CAD build for the part. Positions are in the model's coordinates, mm. A direction names the side the tool comes from. Give positions to 0.01 mm unless a question says otherwise; leave off trailing zeros. Order: outer loops, then holes, each group sorted by start corner. A loop starts at its lowest first (then second) coordinate and runs counter-clockwise, first axis right, second up. Notation, with made-up numbers: (39.5, 34.5) -> (65.5, 34.5) arc R15 cw to (65.5, 41.5) -> close; hole circle Ø4 at (-9.75, 54). An arc over 180 degrees is marked (long way). Use one line per item in the form item = value. Start each with the question number.
1) Cut at D-D, the plane x = 169. Give the cut face in (y, z).
2) Mould opens along Y. For faces 1 (the face through (395, -187, 489.296)), 2 (the face through (238, -278, -5.585)) say: pulls with the +Y half, pulls with the -Y half, needs draft (parallel to the pull), parting line crosses it, or undercut.
3) Cut at A-A, the plane z = 162. Give the cut face in (x, y), and give its area (3 significant figures).
4) Cut at B-B, the plane y = -51. Give the cut face in (x, z).
5) Tool access for faces 3 (the face through (49, -31, 22.261)), 4 (the face through (498.351, -326, 260)), 5 (the face through (235, -186, 564.415)): list every direction of +Z, -Z, +X, -X, +Y, -Y with a clear straight run to the whole face (end or side of a thin tool).
6) Drop flat-ended pins along their axis: P1, Ø10, axis at x = 100.5, z = 456, coming from the -Y side; P2, Ø10.5, axis at x = 473, z = 203.5, coming from the +Y side; P3, Ø3, axis at x = 220, z = 343, coming from the +Y side. Give the stop position or say it passes through.
7) Probe line 1 (X direction, y = -195, z = 46.5); line 2 (X direction, y = -248, z = 331); line 3 (X direction, y = -18, z = 507). List the from-to ranges inside material, lowest first.
8) Cut at C-C, the plane x = 60.5. Give the cut face in (y, z), and give its area (3 significant figures).
from build123d import *

# Parameters (mm, degrees)
F0_W      = 524
F0_H      = 604
F0_W_2    = 520
F0_H_2    = 600
F1_DEPTH  = 340
F2_W      = 310
F2_H      = 240
F2_W_2    = 180
F2_H_2    = 110
F2_H_3    = 5
F3_DEPTH  = 600
F2_W_3    = 65
F2_H_4    = 307.9086494446
F4_DEPTH  = 600
F5_DEPTH  = 600
F6_W      = 182.5336068869
F6_H      = 90
F7_DEPTH  = 70
F8_W      = 180
F8_H      = 29.6823031265
F9_DEPTH  = 110
F10_W     = 62.9086494446
F10_H     = 155
F11_DEPTH = 70
F12_DEPTH = 380
F13_W     = 110
F13_H     = 75
F14_DEPTH = 140
F15_W     = 110
F15_H     = 75.1196961854
F16_DEPTH = 140


with BuildPart() as f1:
    # F0 (on Front) → F1 (new body)
    with BuildSketch(Plane.XZ):
        with Locations((238.3513055446, 264.4152384256)):
            Rectangle(F0_W, F0_H)
        with Locations((238.3513055446, 264.4152384256)):
            Rectangle(F0_W_2, F0_H_2, mode=Mode.SUBTRACT)
    extrude(amount=F1_DEPTH)

    # F2 (on face) → F3 (join)
    with BuildSketch(Plane.XY.offset(-35.5847615744)):
        Polygon((-21.6486944554, -307.9086494446), (-21.6486944554, -312.9086494446), (498.3513055446, -312.9086494446), (498.3513055446, -307.9086494446), (463.3513055446, -307.9086494446), (398.3513055446, -307.9086494446), (393.3513055446, -307.9086494446), (83.3513055446, -307.9086494446), (78.3513055446, -307.9086494446), (13.3513055446, -307.9086494446), align=None)
        with Locations((238.3513055446, -187.9086494446)):
            Rectangle(F2_W, F2_H)
        with Locations((238.3513055446, -187.9086494446)):
            Rectangle(F2_W_2, F2_H_2, mode=Mode.SUBTRACT)
        with Locations((238.3513055446, -65.4086494446)):
            Rectangle(F2_W, F2_H_3)
    extrude(amount=F3_DEPTH)

    # F2 (on face) → F4 (join)
    with BuildSketch(Plane.XY.offset(-35.5847615744)):
        with Locations((45.8513055446, -153.9543247223)):
            Rectangle(F2_W_3, F2_H_4)
        with Locations((430.8513055446, -153.9543247223)):
            Rectangle(F2_W_3, F2_H_4)
    extrude(amount=F4_DEPTH)

    # F2 (on face) → F5 (join)
    with BuildSketch(Plane.XY.offset(-35.5847615744)):
        Polygon((78.3513055446, 0), (78.3513055446, -307.9086494446), (83.3513055446, -307.9086494446), (83.3513055446, -67.9086494446), (83.3513055446, -62.9086494446), (83.3513055446, 0), align=None)
        Polygon((393.3513055446, -307.9086494446), (398.3513055446, -307.9086494446), (398.3513055446, 0), (393.3513055446, 0), (393.3513055446, -62.9086494446), (393.3513055446, -67.9086494446), align=None)
    extrude(amount=F5_DEPTH)

    # F6 (on face) → F7 (cut)
    with BuildSketch(Plane.XZ.offset(312.9086494446)):
        with Locations((239.1115501523, 39.4152384256)):
            Rectangle(F6_W, F6_H)
    extrude(amount=-F7_DEPTH, mode=Mode.SUBTRACT)

    # F8 (on face) → F9 (join)
    with BuildSketch(Plane.XZ.offset(132.9086494446)):
        with Locations((238.3513055446, -20.7436100112)):
            Rectangle(F8_W, F8_H)
    extrude(amount=F9_DEPTH)

    # F10 (on face) → F11 (cut)
    with BuildSketch(Plane(origin=(393.3513055446, 0, 0), x_dir=(0, -1, 0), z_dir=(-1, 0, 0))):
        with Locations((31.4543247223, 99.7613327205)):
            Rectangle(F10_W, F10_H)
    extrude(amount=-F11_DEPTH, mode=Mode.SUBTRACT)

    # F10 (on face) → F12 (cut)
    with BuildSketch(Plane(origin=(393.3513055446, 0, 0), x_dir=(0, -1, 0), z_dir=(-1, 0, 0))):
        with Locations((31.4543247223, 99.7613327205)):
            Rectangle(F10_W, F10_H)
    extrude(amount=F12_DEPTH, mode=Mode.SUBTRACT)

    # F13 (on face) → F14 (cut)
    with BuildSketch(Plane.YZ.offset(148.3513055446)):
        with Locations((-187.9086494446, 526.9152384256)):
            Rectangle(F13_W, F13_H)
    extrude(amount=-F14_DEPTH, mode=Mode.SUBTRACT)

    # F15 (on face) → F16 (cut)
    with BuildSketch(Plane(origin=(328.3513055446, 0, 0), x_dir=(0, -1, 0), z_dir=(-1, 0, 0))):
        with Locations((187.9086494446, 526.8553903329)):
            Rectangle(F15_W, F15_H)
    extrude(amount=-F16_DEPTH, mode=Mode.SUBTRACT)


solid = f1.part
Result:
q1.outline = (-340, -37.58) -> (0, -37.58) -> (0, -35.58) -> (-62.91, -35.58) -> (-62.91, 564.42) -> (0, 564.42) -> (0, 566.42) -> (-340, 566.42) -> (-340, 564.42) -> (-312.91, 564.42) -> (-312.91, 84.42) -> (-242.91, 84.42) -> (-242.91, 564.42) -> (-132.91, 564.42) -> (-132.91, -5.9) -> (-242.91, -5.9) -> (-242.91, -5.58) -> (-312.91, -5.58) -> (-312.91, -35.58) -> (-340, -35.58) -> close
q2.face_1 = undercut
q2.face_2 = needs draft
q3.outline = (-23.65, -340) -> (-21.65, -340) -> (-21.65, -312.91) -> (498.35, -312.91) -> (498.35, -340) -> (500.35, -340) -> (500.35, 0) -> (498.35, 0) -> (498.35, -307.91) -> (463.35, -307.91) -> (463.35, -62.91) -> (13.35, -62.91) -> (13.35, -307.91) -> (-21.65, -307.91) -> (-21.65, 0) -> (-23.65, 0) -> close; hole (148.35, -242.91) -> (328.35, -242.91) -> (328.35, -132.91) -> (148.35, -132.91) -> close
q3.area = 94,400 mm²
q4.outline = (-23.65, -37.58) -> (500.35, -37.58) -> (500.35, 566.42) -> (-23.65, 566.42) -> close; hole (-21.65, -35.58) -> (13.35, -35.58) -> (13.35, 22.26) -> (83.35, 22.26) -> (83.35, -35.58) -> (393.35, -35.58) -> (393.35, 22.26) -> (463.35, 22.26) -> (463.35, -35.58) -> (498.35, -35.58) -> (498.35, 564.42) -> (463.35, 564.42) -> (463.35, 177.26) -> (393.35, 177.26) -> (393.35, 564.42) -> (83.35, 564.42) -> (83.35, 177.26) -> (13.35, 177.26) -> (13.35, 564.42) -> (-21.65, 564.42) -> close
q5.face_3 = +Y
q5.face_4 = -Y
q5.face_5 = none
q6.P1 = -312.91
q6.P2 = -307.91
q6.P3 = -62.91
q7.line_1 = -23.65 to -21.65, 13.35 to 148.35, 328.35 to 463.35, 498.35 to 500.35
q7.line_2 = -23.65 to -21.65, 13.35 to 463.35, 498.35 to 500.35
q7.line_3 = -23.65 to -21.65, 13.35 to 83.35, 393.35 to 463.35, 498.35 to 500.35
q8.outline = (-340, -37.58) -> (0, -37.58) -> (0, 22.26) -> (-62.91, 22.26) -> (-62.91, 177.26) -> (0, 177.26) -> (0, 566.42) -> (-340, 566.42) -> (-340, 564.42) -> (-312.91, 564.42) -> (-312.91, -35.58) -> (-340, -35.58) -> close; hole (-242.91, 489.42) -> (-132.91, 489.42) -> (-132.91, 564.42) -> (-242.91, 564.42) -> close
q8.area = 171,000 mm²
